Can you work these out from the model? Positions are in its coordinate system, mm. A direction names the side the tool comes from. Give positions to 0.01 mm unless a question says otherwise; leave off trailing zeros. Loops run counter-clockwise (first coordinate to the right, second up) from the corner with the lowest first, then second, coordinate; pieces in that order, holes last. Notation, with made-up numbers: (76.25, 61.5) -> (105.25, 61.5) arc R20 ccw to (105.25, 71.5) -> close; hole circle Ø1 at (22, 75.5). An arc over 180 degrees is marked (long way). Return JSON: item names as keys, results as strings. Group by question number.
Q1. Suppose I cut it at B-B, the plane x = 0. Please give me the cut outline in (y, z) (3 decimals).
Q2. Suppose I cut it at A-A, the plane z = 0. Please give me the cut outline in (x, y) (3 decimals).
Q3. Which directions (+Z, -Z, +X, -X, +Y, -Y) give clear straight access to the entire face, cutting with the end or side of a thin tool? Please do faces 1 (the cylindrical face through (-2.17, 1.03, 9.76)), 2 (the flat face through (4, 2.46, -8)).
Q4. Suppose I cut it at C-C, the plane y = 1.2. Please give me the cut outline in (x, z), and give its area (3 significant figures).
Q5. Will these pins go through, and if not, where does the flat tip stop? pin 1 (4 mm diameter, centred on x = -6, z = 6.5, fed in from -Y); pin 2 (1 mm diameter, centred on x = 2, y = 1, fed in from +Z).
Q6. I need wall thicknesses on line 1 along X through (y, z) = (2.6, 1.5); line 2 along X through (y, z) = (0.7, 4.5); line 3 along Z through (x, y) = (-3.75, 0.7). Which ranges of each line are inside material? Lowest first, please. Write a range as [from, to].
```python
from build123d import *

# Parameters (mm, degrees)
FILLET1_R = 0.635
FILLET2_R = 0.254


with BuildPart() as part:
    # Sketch1 → Revolve1 (revolve)
    with BuildSketch(Plane.XY):
        Polygon((0, 0), (0, 3.2), (8.75, 3.2), (8.75, 2.46), (10, 2.46), (10, 0), align=None)
    revolve(axis=Axis((0, 0, 0), (0, 1, 0)))

    # Fillet1
    fillet1_edges = [part.edges().sort_by_distance(p)[0] for p in [
        (-10, 2.46, 0),
        (-8.75, 3.2, 0),
    ]]
    fillet(fillet1_edges, radius=FILLET1_R)

    # Fillet2
    fillet2_edges = [part.edges().sort_by_distance(p)[0] for p in [
        (-10, 0, 0),
    ]]
    fillet(fillet2_edges, radius=FILLET2_R)


solid = part.part
```
Ans:
{
 "1": {"outline": "(0, -9.746) arc R0.254 ccw to (0.254, -10) -> (1.825, -10) arc R0.635 ccw to (2.46, -9.365) -> (2.46, -8.75) -> (2.565, -8.75) arc R0.635 ccw to (3.2, -8.115) -> (3.2, 8.115) arc R0.635 ccw to (2.565, 8.75) -> (2.46, 8.75) -> (2.46, 9.365) arc R0.635 ccw to (1.825, 10) -> (0.254, 10) arc R0.254 ccw to (0, 9.746) -> close"},
 "2": {"outline": "(-10, 0.254) arc R0.254 ccw to (-9.746, 0) -> (9.746, 0) arc R0.254 ccw to (10, 0.254) -> (10, 1.825) arc R0.635 ccw to (9.365, 2.46) -> (8.75, 2.46) -> (8.75, 2.565) arc R0.635 ccw to (8.115, 3.2) -> (-8.115, 3.2) arc R0.635 ccw to (-8.75, 2.565) -> (-8.75, 2.46) -> (-9.365, 2.46) arc R0.635 ccw to (-10, 1.825) -> close"},
 "3": {"face 1": "+Y, -Y", "face 2": "+Y"},
 "4": {"outline": "circle Ø20 at (0, 0)", "area": "314 mm^2"},
 "5": {"pin 1": "stops at y = 0", "pin 2": "stops at z = 9.89"},
 "6": {"line 1": "x = [-8.62, 8.62]", "line 2": "x = [-8.93, 8.93]", "line 3": "z = [-9.27, 9.27]"}
}
